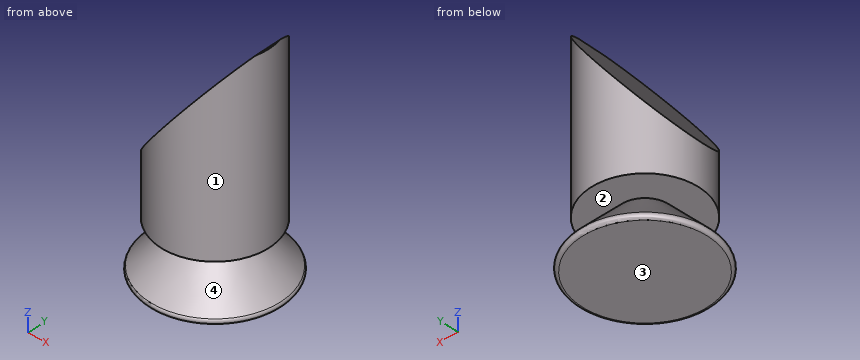
from build123d import *

# Parameters (mm, degrees)
F3_DEPTH = 18.7
F4_R     = 0.714298


with BuildPart() as f1:
    # F0 (on Front) → F1 (revolve)
    with BuildSketch(Plane.XZ):
        Polygon((-15.42939, 0), (0, 0), (0, 50.195612), (-11.82252, 50.195612), (-11.82252, 10.720421), (-5.209924, 10.720421), align=None)
    revolve(axis=Axis((0, 0, 25.097806), (0, 0, -1)))

    # F2 (on Front) → F3 (cut, symmetric)
    with BuildSketch(Plane.XZ):
        Polygon((-17.032443, 13.125001), (14.227101, 53.802483), (-17.032443, 55.806302), align=None)
    extrude(amount=F3_DEPTH, both=True, mode=Mode.SUBTRACT)

    # F4
    f4_edges = [f1.edges().sort_by_distance(p)[0] for p in [
        (15.42939, 0, 0),
    ]]
    fillet(f4_edges, radius=F4_R)


solid = f1.part
CAD build for the part. Positions are in the model's coordinates, mm. Face numbers are marked on the shaded views. A direction names the side the tool comes from. Give positions to 0.01 mm unless a question says otherwise; leave off trailing zeros. Order: outer loops, then holes, each group sorted by start corner. A loop starts at its lowest first (then second) coordinate and runs counter-clockwise, first axis right, second up. Notation, with made-up numbers: (-10.5, 88.5) - (15.5, 88.5) arc R31 cw to (15.5, 113.5) - close; hole circle Ø2 at (37.5, 44). An arc over 180 degrees is marked (long way). Answer in a Markdown table with one row per item.
1. Saw through at A-A, the plane y = 0. Give the cut face in (x, z).
Data:
| item | result |
|---|---|
| outline | (-14.28, 1.21) arc R0.71 ccw to (-13.76, 0) - (13.76, 0) arc R0.71 ccw to (14.28, 1.21) - (5.21, 10.72) - (11.82, 10.72) - (11.82, 50.2) - (11.46, 50.2) - (-11.82, 19.9) - (-11.82, 10.72) - (-5.21, 10.72) - close |
2. Pull direction Z, two halves, no side cores. Call the marked faces 3 and 4: pulls with the +Z half, pulls with the -Z half, needs draft (parallel to the pull), parting line crosses it, or undercut.
Data:
| item | result |
|---|---|
| face 3 | pulls with the -Z half |
| face 4 | undercut |
3. Saw through at D-D, the plane z = 47. Give the cut face in (x, y).
Data:
| item | result |
|---|---|
| outline | (9, -7.67) arc R11.82 ccw to (9, 7.67) - close |
4. Flat gauge pins, fed straight in: pin 1 (1.5 mm diameter, centred on y = 8, z = 35, fed in from +X); pin 2 (10 mm diameter, centred on x = 0.5, y = -10.5, fed in from +Z); pin 3 (1.5 mm diameter, centred on x = 1.5, z = 19, fed in from +Y); pin 4 (7 mm diameter, centred on x = -1, y = 3.5, fed in from -Z). Where does each tip first touch, or does it go through?
Data:
| item | result |
|---|---|
| pin 1 | stops at x = 9.34 |
| pin 2 | stops at z = 42.45 |
| pin 3 | stops at y = 11.8 |
| pin 4 | stops at z = 0 |
5. Saw through at C-C, the plane z = 22.5. Give the cut face in (x, y), plus the area to 3 significant figures.
Data:
| item | result |
|---|---|
| outline | (-9.83, -6.57) arc R11.82 ccw (long way) to (-9.83, 6.57) - close |
| area | 421 mm² |
6. Tool access for the marked faces 1 and 2: list every direction of +Z, -Z, +X, -X, +Y, -Y with a clear straight run to the whole face (end or side of a thin tool).
Data:
| item | result |
|---|---|
| face 1 | +Z |
| face 2 | none |
7. Saw through at B-B, the plane x = 0. Give the cut face in (y, z), plus the area to 3 significant figures.
Data:
| item | result |
|---|---|
| outline | (-14.28, 1.21) arc R0.71 ccw to (-13.76, 0) - (13.76, 0) arc R0.71 ccw to (14.28, 1.21) - (5.21, 10.72) - (11.82, 10.72) - (11.82, 35.29) - (-11.82, 35.29) - (-11.82, 10.72) - (-5.21, 10.72) - close |
| area | 801 mm² |
8. Probe probe 1 along Z at (x, y) = (2.75, 10.75); probe 2 along Z at (x, y) = (5, 4.5); probe 3 along Z at (x, y) = (2.5, 3.75). List the from-to ranges inside material, lowest first. Write a range as [from, to].
Data:
| item | result |
|---|---|
| probe 1 | z = [0, 4.55], [10.72, 38.87] |
| probe 2 | z = [0, 9.13], [10.72, 41.8] |
| probe 3 | z = [0, 38.54] |
